Build history of the part. All positions in model axes, mm. A direction names the side the tool comes from. Round coordinates to 2 decimals unless told otherwise and drop trailing zeros. Order: outer loops, then holes, each group sorted by start corner. A loop starts at its lowest first (then second) coordinate and runs counter-clockwise, first axis right, second up. Notation, with made-up numbers: (-11.5, -38) -> (-3.5, -38) arc R17 ccw to (-3.5, -8) -> close; hole circle Ø3 at (53, 70). An arc over 180 degrees is marked (long way). Answer as CSV lines item,"result". Start each with the question number.
Autodesk Inventor part; units mm, degrees
ref_plane "YZ Plane" through (0, 0, 0) normal (1, 0, 0) x (0, 1, 0)
ref_plane "XZ Plane" through (0, 0, 0) normal (0, 1, 0) x (-1, 0, 0)
ref_plane "XY Plane" through (0, 0, 0) normal (0, 0, 1) x (1, 0, 0)
sketch "Sketch1" plane through (0, 0, 0) normal (0, 0, 1) x (1, 0, 0)
  line L0 (0, 0) -> (25.4, 0)
  line L1 (25.4, 0) -> (25.4, 25.4)
  line L2 (25.4, 25.4) -> (0, 25.4)
  line L3 (0, 25.4) -> (0, 0)
  line L4 (1.5875, 23.8125) -> (23.8125, 23.8125)
  line L5 (23.8125, 23.8125) -> (23.8125, 1.5875)
  line L6 (23.8125, 1.5875) -> (1.5875, 1.5875)
  line L7 (1.5875, 1.5875) -> (1.5875, 23.8125)
  dimension "d0" = 25.4
  dimension "d1" = 25.4
  dimension "d4" = 1.5875
extrude "Extrusion1" add sketch "Sketch1" against normal blind 25.4 contours L3 L2 L1 L0 | L4 L5 L6 L7
extrude "Extrusion2" add sketch "Sketch1" along normal blind 25.4 contours L4 L5 L6 L7
sketch "Sketch2" plane through (25.4, 0, 0) normal (1, 0, 0) x (0, 0, -1)
  line L0 (25.4, 0) -> (25.4, 25.4)
  line L1 (0, 25.4) -> (25.4, 25.4)
  line L2 (0, 0) -> (0, 25.4)
  line L3 (0, 0) -> (25.4, 0)
  line L4 (23.8125, 23.8125) -> (23.8125, 1.5875)
  line L5 (23.8125, 1.5875) -> (1.5875, 1.5875)
  line L6 (1.5875, 1.5875) -> (1.5875, 23.8125)
  line L7 (1.5875, 23.8125) -> (23.8125, 23.8125)
  dimension "d8" = 1.5875
sketch "Sketch3" plane through (0, 25.4, 0) normal (0, 1, 0) x (1, 0, 0)
  line L0 (25.4, 25.4) -> (0, 25.4)
  line L1 (0, 0) -> (0, 25.4)
  line L2 (25.4, 0) -> (0, 0)
  line L3 (25.4, 0) -> (25.4, 25.4)
  line L4 (1.5875, 23.8125) -> (23.8125, 23.8125)
  line L5 (23.8125, 23.8125) -> (23.8125, 1.5875)
  line L6 (23.8125, 1.5875) -> (1.5875, 1.5875)
  line L7 (1.5875, 1.5875) -> (1.5875, 23.8125)
  dimension "d9" = 1.5875
extrude "Extrusion3" add sketch "Sketch2" along normal blind 25.4 contours L4 L5 L6 L7
extrude "Extrusion4" add sketch "Sketch3" along normal blind 25.4 contours L4 L5 L6 L7
sketch "Sketch4" plane through (0, 0, 0) normal (-1, 0, 0) x (0, 0, 1)
  line L0 (-25.4, 25.4) -> (-25.4, 0)
  line L1 (0, 0) -> (-25.4, 0)
  line L2 (0, 25.4) -> (0, 0)
  line L3 (0, 25.4) -> (-25.4, 25.4)
  line L4 (-23.8125, 23.8125) -> (-23.8125, 1.5875)
  line L5 (-23.8125, 1.5875) -> (-1.5875, 1.5875)
  line L6 (-1.5875, 1.5875) -> (-1.5875, 23.8125)
  line L7 (-1.5875, 23.8125) -> (-23.8125, 23.8125)
  dimension "d15" = 1.5875
extrude "Extrusion5" add sketch "Sketch4" along normal blind 25.4 contours L7 L6 L5 L4
sketch "Sketch5" plane through (0, 0, -25.4) normal (0, 0, -1) x (-1, 0, 0)
  line L0 (-25.4, 0) -> (-25.4, 25.4)
  line L1 (0, 0) -> (-25.4, 0)
  line L2 (0, 25.4) -> (0, 0)
  line L3 (-25.4, 25.4) -> (0, 25.4)
  line L4 (-1.5875, 23.8125) -> (-1.5875, 1.5875)
  line L5 (-1.5875, 1.5875) -> (-23.8125, 1.5875)
  line L6 (-23.8125, 1.5875) -> (-23.8125, 23.8125)
  line L7 (-23.8125, 23.8125) -> (-1.5875, 23.8125)
  dimension "d18" = 1.5875
extrude "Extrusion6" add sketch "Sketch5" along normal blind 25.4 contours L4 L5 L6 L7
sketch "Sketch6" plane through (0, 0, 0) normal (0, -1, 0) x (1, 0, 0)
  line L0 (0, -25.4) -> (25.4, -25.4)
  line L1 (25.4, 0) -> (25.4, -25.4)
  line L2 (0, 0) -> (25.4, 0)
  line L3 (0, 0) -> (0, -25.4)
  line L4 (23.8125, -23.8125) -> (1.5875, -23.8125)
  line L5 (1.5875, -23.8125) -> (1.5875, -1.5875)
  line L6 (1.5875, -1.5875) -> (23.8125, -1.5875)
  line L7 (23.8125, -1.5875) -> (23.8125, -23.8125)
  dimension "d21" = 1.5875
extrude "Extrusion7" add sketch "Sketch6" along normal blind 25.4 contours L4 L5 L6 L7
sketch "Sketch7" plane through (0, 1.5875, -23.8125) normal (0, -1, 0) x (1, 0, 0)
  line L0 (0, 22.225) -> (0, 0)
  line L1 (0, 23.8125) -> (25.4, 23.8125)
  line L2 (25.4, 23.8125) -> (25.4, -1.5875)
  point P0 (-12.7, 11.1125)
  point P1 (38.1, 11.1125)
  point P2 (12.6993, -14.2875)
  point P3 (12.7, 36.5125)
  dimension "d24" = 12.7
  dimension "d25" = 50.8
  dimension "d26" = 12.7
  dimension "d27" = 12.7
  dimension "d28" = 12.7
hole "Hole1" at (-12.7, 1.5875, -12.7) at (38.1, 1.5875, -12.7) at (12.6993, 1.5875, -38.1) at (12.7, 1.5875, 12.7) direction (0, 1, 0) diameter 6.35 depth 25.4 tip angle 118
sketch "Sketch8" plane through (1.5875, 0, -23.8125) normal (-1, 0, 0) x (0, 0, 1)
  line L0 (0, -25.4) -> (22.225, -25.4)
  line L1 (0, 0) -> (0, -25.4)
  point P0 (23.8125, 0)
  point P1 (11.1125, -12.7)
  point P2 (11.1125, 38.1)
  dimension "d36" = 50.8
  dimension "d37" = 12.7
  dimension "d38" = 11.1125
hole "Hole2" at (1.5875, -12.7, -12.7) at (1.5875, 38.1, -12.7) direction (1, 0, 0) diameter 6.35 depth 25.4 tip angle 118
sketch "Sketch9" plane through (1.5875, 0, -1.5875) normal (0, 0, 1) x (1, 0, 0)
  line L0 (0, -25.4) -> (22.225, -25.4)
  point P0 (-1.5875, 0)
  point P1 (11.1125, -12.7)
  point P2 (11.1125, 38.1)
  dimension "d46" = 50.8
  dimension "d47" = 12.7
hole "Hole3" at (12.7, -12.7, -1.5875) at (12.7, 38.1, -1.5875) direction (0, 0, -1) diameter 6.35 depth 25.4 tip angle 118
properties part number "6-way corner"
Q1. Slice it at B-B, the plane x = 38.1. Write the cut outline in (y, z) (1 decimal), plus the area to 3 significant figures.
Q2. Slice it at D-D, the plane z = -18. Count the separate pieces of the cut face and the enclosed holes in it, plus the area to 3 significant figures.
Q3. Slice it at A-A, the plane z = -38.1. Write the cut outline in (x, y), plus the area to 3 significant figures.
Q4. Probe L1, parallel to Y at x = 16.5, z = -12.7 (3 decimals); L2, parallel to Z at x = 11, y = 9.5. List the from-to ranges inside material, lowest first.
Q5. Which spindle directions (+Z, -Z, +X, -X, +Y, -Y) get a long thin tool onto all of the face, cutting with end or side? Do faces 1 (the face through (-15.3, 1.588, -15.3)), 2 (the face through (15, 23.812, -35)), 3 (the face through (23.812, 35, -15)), 4 (the face through (38, 13, -1.588)). Say none if no direction does.
Q6. Slice it at C-C, the plane y = -12.7. Write the cut outline in (x, z) (1 decimal).
Q7. Two-plate mould, pull along Y, no slides. Class faces 5 (the face through (5.987, 35.423, -10.993)), 6 (the face through (15.3, 1.588, 15.3)), 7 (the face through (1.588, 13, 13)): +Y half, -Y half, draft (parallel to the pull), parting line (faces both ways), or undercut.
Q8. Flat gauge pins, fed straight in: pin 1 Ø24.5 at (y, z) = (17, -43.5) entering from +X; pin 2 Ø1 at (x, z) = (-5, 0) entering from +Y; pin 3 Ø8.5 at (x, z) = (12.7, 12.7) entering from +Y; pin 4 Ø8 at (x, z) = (40.5, -1.5) entering from -Y. Where does each tip first touch, or does it go through?
Solutions:
1,outline,"(1.6, -23.8) -> (23.8, -23.8) -> (23.8, -15.9) -> (1.6, -15.9) -> close; (1.6, -9.5) -> (23.8, -9.5) -> (23.8, -1.6) -> (1.6, -1.6) -> close"
1,area,"353 mm2"
2,separate pieces,"1"
2,enclosed holes,"2"
2,area,"2,840 mm2"
3,outline,"(1.59, 1.59) -> (9.52, 1.59) -> (9.52, 23.81) -> (1.59, 23.81) -> close; (15.87, 1.59) -> (23.81, 1.59) -> (23.81, 23.81) -> (15.87, 23.81) -> close"
3,area,"353 mm2"
4,L1,"y = -25.4 to -15.875, -9.525 to 34.925, 41.275 to 50.8"
4,L2,"z = -50.8 to -40.78, -35.42 to 10.02, 15.38 to 25.4"
5,face 1,"+Z, -Z, -X, -Y"
5,face 2,"-Z, +X, -X, +Y"
5,face 3,"+Z, -Z, +X, +Y"
5,face 4,"+Z, +X, +Y, -Y"
6,outline,"(1.6, -23.8) -> (9.5, -23.8) -> (9.5, -15.9) -> (1.6, -15.9) -> close; (1.6, -9.5) -> (9.5, -9.5) -> (9.5, -1.6) -> (1.6, -1.6) -> close; (15.9, -23.8) -> (23.8, -23.8) -> (23.8, -15.9) -> (15.9, -15.9) -> close; (15.9, -9.5) -> (23.8, -9.5) -> (23.8, -1.6) -> (15.9, -1.6) -> close"
7,face 5,"undercut"
7,face 6,"-Y half"
7,face 7,"draft"
8,pin 1,"stops at x = 23.81"
8,pin 2,"passes through"
8,pin 3,"stops at y = 23.81"
8,pin 4,"stops at y = 1.59"
